```python
from build123d import *

# Parameters (mm, degrees)
SKETCH1_R           = 1.5875
BOSS_EXTRUDE1_DEPTH = 3.175


with BuildPart() as part:
    # Sketch1 → Boss-Extrude1 (new body)
    with BuildSketch(Plane.XY):
        Polygon((0, 0), (6.35, 0), (6.35, -3.175), (19.05, -3.175), (19.05, 0), (31.75, 0), (31.75, -3.175), (44.45, -3.175), (44.45, 0), (50.8, 0), (50.8, 106.875), (0, 106.875), align=None)
        with Locations((11.1125, 97.35)):
            Circle(SKETCH1_R, mode=Mode.SUBTRACT)
        with Locations((11.1125, 69.85)):
            Circle(SKETCH1_R, mode=Mode.SUBTRACT)
        with Locations((40.1125, 97.35)):
            Circle(SKETCH1_R, mode=Mode.SUBTRACT)
        with Locations((40.1125, 69.85)):
            Circle(SKETCH1_R, mode=Mode.SUBTRACT)
    extrude(amount=BOSS_EXTRUDE1_DEPTH)


solid = part.part
```
Could you check a few things on this model? Use its own coordinates, in mm. A direction names the side the tool comes from. Coordinates: 2 decimals unless noted, no trailing zeros. Write each loop counter-clockwise with the first axis right and the second up, starting at its lowest first coordinate (ties: lowest second). Pieces come first, ordered by that corner, then holes. Notation, with made-up numbers: (-24.5, -7.75) -> (10.5, -7.75) arc R15 cw to (10.5, 10.25) -> close; hole circle Ø2 at (-16.75, -3.5). An arc over 180 degrees is marked (long way). One line per question, with ' | ' between items. Start each with the question number.
1. For faces 5 (the face through (48, 0, 2)), 6 (the face through (31.75, -2, 2)), 7 (the face through (12.627, 70.327, 1.565)), 8 (the face through (13, -3.175, 2)), 9 (the face through (3, 0, 2)), which set-ups out of +Z, -Z, +X, -X, +Y, -Y let a thin tool reach every point of the face, with its end or its side?
2. If we section it at B-B (y = 97.35): Please give me the cut outline in (x, z) (3 decimals).
3. If we section it at A-A (z = 0.6): Count the separate pieces of the cut face and the enclosed holes in it, and give its area (3 significant figures).
4. Please list where these lines run through material, in increasing order: line 1 along X through (y, z) = (69.85, 1.6) (3 decimals); line 2 along Y through (x, z) = (10, 0.7) (3 decimals); line 3 along Y through (x, z) = (22, 1.15) (3 decimals).
5. Will these pins go through, and if not, where does the flat tip stop? P1, Ø1.9, axis at x = 11.11, y = 97.35, coming from the +Z side; P2, Ø1, axis at y = -1.5, z = 2, coming from the -X side; P3, Ø1.6, axis at x = 2, z = 1, coming from the -Y side.
6. Thinking about a two-plate mould opening in X: for faces 1 (the face through (10.906, 98.924, 1.565)), 2 (the face through (50.8, 53, 2)), 3 (the face through (25, 0, 2)), 4 (the face through (0, 54, 2)), which applies, pulls with the +X half, pulls with the -X half, needs draft (parallel to the pull), parting line crosses it, or undercut?
7. If we section it at C-C (x = 20.5): Please give me the cut outline in (y, z) (3 decimals), and give its area (3 significant figures).
Return value:
1) face 5: +Z, -Z, +X, -Y | face 6: +Z, -Z, -Y | face 7: +Z, -Z | face 8: +Z, -Z, +X, -X, -Y | face 9: +Z, -Z, -X, -Y
2) outline: (0, 0) -> (9.525, 0) -> (9.525, 3.175) -> (0, 3.175) -> close; (12.7, 0) -> (38.525, 0) -> (38.525, 3.175) -> (12.7, 3.175) -> close; (41.7, 0) -> (50.8, 0) -> (50.8, 3.175) -> (41.7, 3.175) -> close
3) separate pieces: 1 | enclosed holes: 4 | area: 5,480 mm²
4) line 1: x = 0 to 9.525, 12.7 to 38.525, 41.7 to 50.8 | line 2: y = -3.175 to 68.718, 70.982 to 96.218, 98.482 to 106.875 | line 3: y = 0 to 106.875
5) P1: passes through | P2: stops at x = 6.35 | P3: stops at y = 0
6) face 1: undercut | face 2: pulls with the +X half | face 3: undercut | face 4: pulls with the -X half
7) outline: (0, 0) -> (106.875, 0) -> (106.875, 3.175) -> (0, 3.175) -> close | area: 339 mm²
